from build123d import *

# Parameters (mm, degrees)
SKETCH_1_W          = 81
SKETCH_1_H          = 61
EXTRUDE_1_DEPTH     = 23
SHELL_1_T           = -2
SKETCH_2_R          = 2.15
EXTRUDE_3_DEPTH     = 4
SKETCH_3_R          = 1.9
CUT_EXTRUDE_1_DEPTH = 2
SKETCH_4_R          = 2.7
SKETCH_4_R_2        = 1.9
CUT_EXTRUDE_2_DEPTH = 0.8
SKETCH_5_W          = 31
SKETCH_5_H          = 12
SKETCH_5_W_2        = 7.1
SKETCH_5_H_2        = 8
CUT_EXTRUDE_3_DEPTH = 2
SKETCH_6_W          = 14
SKETCH_6_H          = 11
CUT_EXTRUDE_4_DEPTH = 2
SKETCH_7_W          = 14
SKETCH_7_H          = 11
CUT_EXTRUDE_5_DEPTH = 2


with BuildPart() as part:
    # 草图1 → 凸台-拉伸1 (new body)
    with BuildSketch(Plane(origin=(0, 0, 0), x_dir=(1, 0, 0), z_dir=(0, 1, 0))):
        Rectangle(SKETCH_1_W, SKETCH_1_H)
    extrude(amount=EXTRUDE_1_DEPTH)

    # 抽壳1
    shell_1_openings = [part.faces().sort_by_distance(p)[0] for p in [
        (0, 23, 0),
    ]]
    offset(amount=SHELL_1_T, openings=shell_1_openings, kind=Kind.INTERSECTION)

    # 草图2 → 凸台-拉伸3 (add)
    with BuildSketch(Plane.XZ):
        with BuildLine():
            Line((-45.5, 5), (-40.5, 5))
            Line((-40.5, 5), (-40.5, -5))
            Line((-40.5, -5), (-45.5, -5))
            ThreePointArc((-45.5, -5), (-50.5, 0), (-45.5, 5))
        make_face()
        with Locations((-45.5, 0)):
            Circle(SKETCH_2_R, mode=Mode.SUBTRACT)
        with BuildLine():
            Line((40.5, -5), (45.5, -5))
            ThreePointArc((45.5, -5), (50.5, 0), (45.5, 5))
            Line((45.5, 5), (40.5, 5))
            Line((40.5, 5), (40.5, -5))
        make_face()
        with Locations((45.5, 0)):
            Circle(SKETCH_2_R, mode=Mode.SUBTRACT)
    extrude(amount=-EXTRUDE_3_DEPTH)

    # 草图3 → 切除-拉伸1 (cut)
    with BuildSketch(Plane(origin=(0, 0, 0), x_dir=(1, 0, 0), z_dir=(0, 1, 0))):
        with Locations((-34.45, -24.55)):
            Circle(SKETCH_3_R)
        with Locations((-34.45, 24.55)):
            Circle(SKETCH_3_R)
        with Locations((34.45, 24.55)):
            Circle(SKETCH_3_R)
        with Locations((34.45, -24.55)):
            Circle(SKETCH_3_R)
    extrude(amount=CUT_EXTRUDE_1_DEPTH, mode=Mode.SUBTRACT)

    # 草图4 → 切除-拉伸2 (cut)
    with BuildSketch(Plane(origin=(0, 0, 0), x_dir=(1, 0, 0), z_dir=(0, 1, 0))):
        with Locations((-34.45, -24.55)):
            Circle(SKETCH_4_R)
        with Locations((-34.45, -24.55)):
            Circle(SKETCH_4_R_2, mode=Mode.SUBTRACT)
        with Locations((-34.45, 24.55)):
            Circle(SKETCH_4_R)
        with Locations((-34.45, 24.55)):
            Circle(SKETCH_4_R_2, mode=Mode.SUBTRACT)
        with Locations((34.45, 24.55)):
            Circle(SKETCH_4_R)
        with Locations((34.45, 24.55)):
            Circle(SKETCH_4_R_2, mode=Mode.SUBTRACT)
        with Locations((34.45, -24.55)):
            Circle(SKETCH_4_R)
        with Locations((34.45, -24.55)):
            Circle(SKETCH_4_R_2, mode=Mode.SUBTRACT)
    extrude(amount=CUT_EXTRUDE_2_DEPTH, mode=Mode.SUBTRACT)

    # 草图5 → 切除-拉伸3 (cut)
    with BuildSketch(Plane(origin=(40.5, 0, 0), x_dir=(0, 0, -1), z_dir=(1, 0, 0))):
        with Locations((-5.3, 17)):
            Rectangle(SKETCH_5_W, SKETCH_5_H)
        with Locations((15.45, 16)):
            Rectangle(SKETCH_5_W_2, SKETCH_5_H_2)
    extrude(amount=-CUT_EXTRUDE_3_DEPTH, mode=Mode.SUBTRACT)

    # 草图6 → 切除-拉伸4 (cut)
    with BuildSketch(Plane(origin=(0, 0, -30.5), x_dir=(-1, 0, 0), z_dir=(0, 0, -1))):
        with Locations((9.5, 11.5)):
            Rectangle(SKETCH_6_W, SKETCH_6_H)
    extrude(amount=-CUT_EXTRUDE_4_DEPTH, mode=Mode.SUBTRACT)

    # 草图7 → 切除-拉伸5 (cut)
    with BuildSketch(Plane.ZY.offset(40.5)):
        with Locations((11.3, 16)):
            Rectangle(SKETCH_7_W, SKETCH_7_H)
        with Locations((-7.3, 16)):
            Rectangle(SKETCH_7_W, SKETCH_7_H)
    extrude(amount=-CUT_EXTRUDE_5_DEPTH, mode=Mode.SUBTRACT)


solid = part.part
Design review of the part built by this model. Coordinates are the model's own, in mm. A direction names the side the tool comes from. Coordinates: 2 decimals unless noted, no trailing zeros. Write each loop counter-clockwise with the first axis right and the second up, starting at its lowest first coordinate (ties: lowest second). Pieces come first, ordered by that corner, then holes. Notation, with made-up numbers: (-36.75, 87.5) - (-18.75, 87.5) arc R37 ccw to (-18.75, 126.5) - close; hole circle Ø6 at (37.5, 73.25). An arc over 180 degrees is marked (long way). One line per item, written item: value.
1) To check wall thickness, follow probe 1 along X at (y, z) = (0.55, -24.55); probe 2 along Z at (x, y) = (34.45, 0.65); probe 3 along Z at (x, y) = (-34.45, 1.55). State the ranges of each line that lie inside material, in increasing order.
Answer sheet:
probe 1: x = -40.5 to -37.15, -31.75 to 31.75, 37.15 to 40.5
probe 2: z = -30.5 to -27.25, -21.85 to 21.85, 27.25 to 30.5
probe 3: z = -30.5 to -26.45, -22.65 to 22.65, 26.45 to 30.5
2) Add section D-D (z = 14.5). State the section outline as (x, y) points.
Answer sheet:
outline: (-40.5, 0) - (40.5, 0) - (40.5, 11) - (38.5, 11) - (38.5, 2) - (-38.5, 2) - (-38.5, 10.5) - (-40.5, 10.5) - close; (-40.5, 21.5) - (-38.5, 21.5) - (-38.5, 23) - (-40.5, 23) - close
3) Add section C-C (y = 14.25). State the section outline as (x, z) points, plus the area to 3 significant figures.
Answer sheet:
outline: (-40.5, -30.5) - (-16.5, -30.5) - (-16.5, -28.5) - (-38.5, -28.5) - (-38.5, -14.3) - (-40.5, -14.3) - close; (-40.5, -0.3) - (-38.5, -0.3) - (-38.5, 4.3) - (-40.5, 4.3) - close; (-40.5, 18.3) - (-38.5, 18.3) - (-38.5, 28.5) - (38.5, 28.5) - (38.5, 20.8) - (40.5, 20.8) - (40.5, 30.5) - (-40.5, 30.5) - close; (-2.5, -30.5) - (40.5, -30.5) - (40.5, -19) - (38.5, -19) - (38.5, -28.5) - (-2.5, -28.5) - close; (38.5, -11.9) - (40.5, -11.9) - (40.5, -10.2) - (38.5, -10.2) - close
area: 392 mm2
4) Insertion check: pin 1 (1.6 mm diameter, centred on x = 34, z = -23.5, fed in from -Y); pin 2 (10 mm diameter, centred on y = 4.5, z = 20.5, fed in from +X); pin 3 (11 mm diameter, centred on x = -46.5, z = -1.5, fed in from +Y). Each pin has a flat end and moves straight along its axis. Give the tip position at first contact, or say it passes through.
Answer sheet:
pin 1: stops at y = 0.8
pin 2: stops at x = 40.5
pin 3: stops at y = 4
5) Add section B-B (z = 24.55). State the section outline as (x, y) points.
Answer sheet:
outline: (-40.5, 0) - (-37.15, 0) - (-37.15, 0.8) - (-36.35, 0.8) - (-36.35, 2) - (-38.5, 2) - (-38.5, 23) - (-40.5, 23) - close; (-32.55, 0.8) - (-31.75, 0.8) - (-31.75, 0) - (31.75, 0) - (31.75, 0.8) - (32.55, 0.8) - (32.55, 2) - (-32.55, 2) - close; (36.35, 0.8) - (37.15, 0.8) - (37.15, 0) - (40.5, 0) - (40.5, 23) - (38.5, 23) - (38.5, 2) - (36.35, 2) - close
6) For faces 3 (the face through (-40, 21.5, -7)), 4 (the face through (-43, 2, 5)), 5 (the face through (36, 0.8, 26)), 6 (the face through (-9, 17, -30)), list the 3-axis set-ups (+Z, -Z, +X, -X, +Y, -Y) from which the entire face can be reached by the end or side of a thin tool; tool diameter is ignored.
Answer sheet:
face 3: -X
face 4: +Z, -X, +Y, -Y
face 5: -Y
face 6: -Z
7) Mouldability with a two-part tool opening along X and no side actions: class faces 1 (the face through (40, 16, -11.9)), 2 (the face through (-1, 12, 28.5)) as +X half, -X half, draft (parallel to the pull), parting line (faces both ways), or undercut.
Answer sheet:
face 1: draft
face 2: undercut
8) Add section A-A (x = -34.45). State the section outline as (y, z) points.
Answer sheet:
outline: (0, -30.5) - (23, -30.5) - (23, -28.5) - (2, -28.5) - (2, -26.45) - (0.8, -26.45) - (0.8, -27.25) - (0, -27.25) - close; (0, -21.85) - (0.8, -21.85) - (0.8, -22.65) - (2, -22.65) - (2, 22.65) - (0.8, 22.65) - (0.8, 21.85) - (0, 21.85) - close; (0, 27.25) - (0.8, 27.25) - (0.8, 26.45) - (2, 26.45) - (2, 28.5) - (23, 28.5) - (23, 30.5) - (0, 30.5) - close
